Check sheet for the modelled part. Datum: model origin and axes. Units: mm. Face numbers are marked on the shaded views. Round coordinates to 2 decimals unless told otherwise and drop trailing zeros. Write each loop counter-clockwise with the first axis right and the second up, starting at its lowest first coordinate (ties: lowest second). Pieces come first, ordered by that corner, then holes.
Item 1: Material ranges on line 1 along Y through (x, z) = (0, 2.5); line 2 along X through (y, z) = (60, 8); line 3 along X through (y, z) = (19, 5.75), recorded low to high.
Item 2: Section check A-A, the plane y = 0. Record the cut outline in (x, z).
Item 3: Section check C-C, the plane x = 64. Record the cut outline in (y, z), plus the area to 3 significant figures.
Item 4: Depth check by flat-ended pin: pin 1 (7 mm diameter, centred on x = 0, y = 78.75, fed in from +Z); pin 2 (4 mm diameter, centred on x = -54.5, z = 4, fed in from -Y); pin 3 (3 mm diameter, centred on x = 8, z = 4, fed in from +Y); pin 4 (1.5 mm diameter, centred on x = 50, z = 4, fed in from -Y). Enter the tip coordinate at first touch or a pass-through.
Item 5: Section check D-D, the plane z = 6.5. Record the cut outline in (x, y).
Item 6: Release check for a two-part mould opening along Z. For the marked faces 1 and 2 record: pulls with the +Z half, pulls with the -Z half, needs draft (parallel to the pull), parting line crosses it, or undercut.
Autodesk Inventor part; units mm, degrees
ref_plane "YZ Plane" through (0, 0, 0) normal (1, 0, 0) x (0, 1, 0)
ref_plane "XZ Plane" through (0, 0, 0) normal (0, 1, 0) x (-1, 0, 0)
ref_plane "XY Plane" through (0, 0, 0) normal (0, 0, 1) x (1, 0, 0)
sketch "スケッチ1" plane through (0, 0, 0) normal (0, 0, 1) x (1, 0, 0)
  circle A0 centre (0, 0) radius 72.5
  circle A1 centre (0, 0) radius 85
  circle A2 centre (0, 0) radius 78.75 construction
  circle A3 centre (0, 78.75) radius 4
  circle A4 centre (78.75, 0) radius 4
  circle A5 centre (0, -78.75) radius 4
  circle A6 centre (-78.75, 0) radius 4
  dimension "d0" = 145
  dimension "d1" = 170
  dimension "d14" = 157.5
  dimension "d15" = 8
  dimension "d16" = 8
  dimension "d17" = 8
  dimension "d18" = 8
extrude "押し出し2" add sketch "スケッチ1" along normal blind 8.5
properties part number "ベアリング 内側"
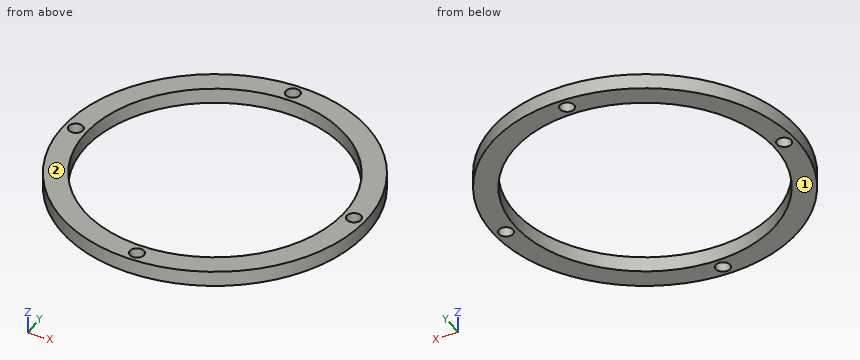
Values found:
1. line 1: y = -85 to -82.75, -74.75 to -72.5, 72.5 to 74.75, 82.75 to 85
1. line 2: x = -60.21 to -40.7, 40.7 to 60.21
1. line 3: x = -82.85 to -69.97, 69.97 to 82.85
2. outline: (-85, 0) - (-82.75, 0) - (-82.75, 8.5) - (-85, 8.5) - close; (-74.75, 0) - (-72.5, 0) - (-72.5, 8.5) - (-74.75, 8.5) - close; (72.5, 0) - (74.75, 0) - (74.75, 8.5) - (72.5, 8.5) - close; (82.75, 0) - (85, 0) - (85, 8.5) - (82.75, 8.5) - close
3. outline: (-55.94, 0) - (-34.06, 0) - (-34.06, 8.5) - (-55.94, 8.5) - close; (34.06, 0) - (55.94, 0) - (55.94, 8.5) - (34.06, 8.5) - close
3. area: 372 mm2
4. pin 1: passes through
4. pin 2: stops at y = -66.85
4. pin 3: stops at y = 84.75
4. pin 4: stops at y = -69.28
5. outline: circle Ø170 at (0, 0); hole circle Ø8 at (-78.75, 0); hole circle Ø145 at (0, 0); hole circle Ø8 at (0, -78.75); hole circle Ø8 at (0, 78.75); hole circle Ø8 at (78.75, 0)
6. face 1: pulls with the -Z half
6. face 2: pulls with the +Z half
